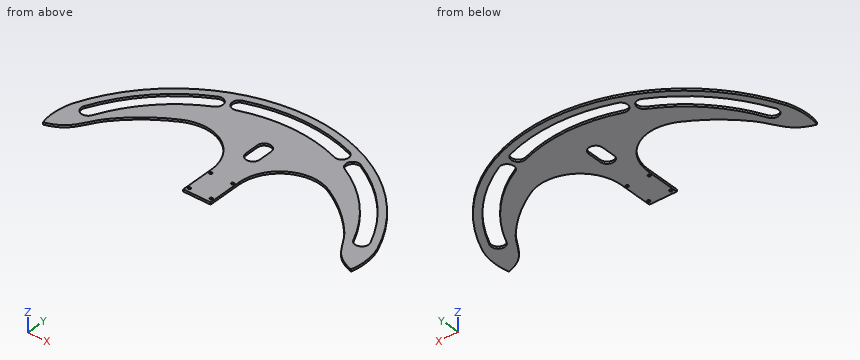
from build123d import *

# Parameters (mm, degrees)
EXTRUDE_2_DEPTH     = 1.6
SKETCH_2_R          = 1
CUT_EXTRUDE_1_DEPTH = 152.556112047


with BuildPart() as part:
    # 草图1 → 凸台-拉伸2 (new body)
    with BuildSketch(Plane.XY):
        with BuildLine():
            Line((-10, 0), (10, 0))
            Line((10, 0), (10, 25))
            ThreePointArc((10, 25), (24.565127337, 50.724787771), (54.117647059, 51.470588235))
            ThreePointArc((54.117647059, 51.470588235), (71.876884233, 39.7703376), (87.177978871, 25))
            add(Edge.make_bspline(
                [(87.177978871, 25), (90.304994573, 21.365241216), (96.247853251, 9.443363931), (103.450341903, 2.775811449), (112.5, 0)],
                knots=[0, 0, 0, 0, 0.44500112, 1, 1, 1, 1], degree=3))
            add(Edge.make_bspline(
                [(111.242977306, 25), (112.528770299, 21.821434652), (115.6681563, 10.742987267), (112.5, 0)],
                knots=[0, 0, 0, 0, 1, 1, 1, 1], degree=3))
            ThreePointArc((111.242977306, 25), (0, 100), (-111.242977306, 25))
            add(Edge.make_bspline(
                [(-111.242977306, 25), (-112.528770299, 21.821434652), (-115.6681563, 10.742987267), (-112.5, 0)],
                knots=[0, 0, 0, 0, 1, 1, 1, 1], degree=3))
            add(Edge.make_bspline(
                [(-87.177978871, 25), (-90.304994573, 21.365241216), (-96.247853251, 9.443363931), (-103.450341903, 2.775811449), (-112.5, 0)],
                knots=[0, 0, 0, 0, 0.44500112, 1, 1, 1, 1], degree=3))
            ThreePointArc((-87.177978871, 25), (-71.876884233, 39.7703376), (-54.117647059, 51.470588235))
            ThreePointArc((-54.117647059, 51.470588235), (-24.565127337, 50.724787771), (-10, 25))
            Line((-10, 25), (-10, 0))
        make_face()
        with BuildLine():
            Line((5, 59.658560997), (5, 49.658560997))
            ThreePointArc((5, 49.658560997), (0, 44.658560997), (-5, 49.658560997))
            Line((-5, 49.658560997), (-5, 59.658560997))
            ThreePointArc((-5, 59.658560997), (0, 64.658560997), (5, 59.658560997))
        make_face(mode=Mode.SUBTRACT)
        with BuildLine():
            ThreePointArc((-52.279803763, 82.046105896), (-83.1008003, 58.999003788), (-104.559607526, 27.051823387))
            ThreePointArc((-104.559607526, 27.051823387), (-102.051823387, 20.440392474), (-95.440392474, 22.948176613))
            ThreePointArc((-95.440392474, 22.948176613), (-75.853125153, 52.10906874), (-47.720196237, 73.146107064))
            ThreePointArc((-47.720196237, 73.146107064), (-45.550000584, 79.875910243), (-52.279803763, 82.046105896))
        make_face(mode=Mode.SUBTRACT)
        with BuildLine():
            ThreePointArc((52.279803763, 82.046105896), (83.1008003, 58.999003788), (104.559607526, 27.051823387))
            ThreePointArc((104.559607526, 27.051823387), (102.051823387, 20.440392474), (95.440392474, 22.948176613))
            ThreePointArc((95.440392474, 22.948176613), (75.853125153, 52.10906874), (47.720196237, 73.146107064))
            ThreePointArc((47.720196237, 73.146107064), (45.550000584, 79.875910243), (52.279803763, 82.046105896))
        make_face(mode=Mode.SUBTRACT)
        with BuildLine():
            ThreePointArc((39.209852822, 87.74587255), (0, 94.658560997), (-39.209852822, 87.74587255))
            ThreePointArc((-39.209852822, 87.74587255), (-42.198553323, 81.337466405), (-35.790147178, 78.348765905))
            ThreePointArc((-35.790147178, 78.348765905), (0, 84.658560997), (35.790147178, 78.348765905))
            ThreePointArc((35.790147178, 78.348765905), (42.198553323, 81.337466405), (39.209852822, 87.74587255))
        make_face(mode=Mode.SUBTRACT)
    extrude(amount=EXTRUDE_2_DEPTH)

    # 草图2 → 切除-拉伸1 (cut, through all)
    with BuildSketch(Plane.XY.offset(1.6)):
        with Locations((-8, 3)):
            Circle(SKETCH_2_R)
        with Locations(Location((8, 3, 0), (0, 0, 180))):
            Circle(SKETCH_2_R)
        with Locations((-8, 22)):
            Circle(SKETCH_2_R)
        with Locations(Location((8, 22, 0), (0, 0, 180))):
            Circle(SKETCH_2_R)
    extrude(amount=-CUT_EXTRUDE_1_DEPTH, mode=Mode.SUBTRACT)


solid = part.part
Could you check a few things on this model? Use its own coordinates, in mm. Give positions to 0.01 mm unless a question says otherwise; leave off trailing zeros. Order: outer loops, then holes, each group sorted by start corner. A loop starts at its lowest first (then second) coordinate and runs counter-clockwise, first axis right, second up. Notation, with made-up numbers: (19.25, -1) -> (47.25, -1) arc R20 cw to (47.25, 29) -> close; hole circle Ø2 at (41, 49.25). An arc over 180 degrees is marked (long way). Answer in a Markdown table with one row per item. Add a question column.
Item 1: Please list where these lines run through material, in increasing order: probe 1 along X at (y, z) = (5, 0.6); probe 2 along Y at (x, z) = (-8, 0.95); probe 3 along X at (y, z) = (50, 0.45).
Item 2: Imagine slicing it at A-A (x = 0). List the corners of the cut face in (y, z) for me.
Item 3: I'm going to push flat-ended pins straight in: P1, Ø12, axis at x = -32, y = 89, coming from the +Z side; P2, Ø0.8, axis at y = 17.5, z = 1, coming from the -X side. Where does each tip first touch, or does it pass through?
Item 4: Imagine slicing it at C-C (y = 34). List the corners of the cut face in (x, z) for me, and give its area (3 significant figures).
Item 5: Imagine slicing it at D-D (z = 1.15). Count the separate pieces of the cut face and the enclosed holes in it, and give its area (3 significant figures).
Item 6: Imagine slicing it at B-B (x = -50). List the corners of the cut face in (y, z) for me.
Result:
| question | item | result |
|---|---|---|
| 1 | probe 1 | -113.55 to -102.06, -10 to 10, 102.06 to 113.55 |
| 1 | probe 2 | 0 to 2, 4 to 21, 23 to 84.35, 94.38 to 99.73 |
| 1 | probe 3 | -97.47 to -90.81, -77.8 to -56.79, -23.42 to -5, 5 to 23.42, 56.79 to 77.8, 90.81 to 97.47 |
| 2 | outline | (0, 0) -> (44.66, 0) -> (44.66, 1.6) -> (0, 1.6) -> close; (64.66, 0) -> (84.66, 0) -> (84.66, 1.6) -> (64.66, 1.6) -> close; (94.66, 0) -> (100, 0) -> (100, 1.6) -> (94.66, 1.6) -> close |
| 3 | P1 | z = 1.6 |
| 3 | P2 | x = -113.29 |
| 4 | outline | (-107.16, 0) -> (-101.15, 0) -> (-101.15, 1.6) -> (-107.16, 1.6) -> close; (-89.65, 0) -> (-78.54, 0) -> (-78.54, 1.6) -> (-89.65, 1.6) -> close; (-11.38, 0) -> (11.38, 0) -> (11.38, 1.6) -> (-11.38, 1.6) -> close; (78.54, 0) -> (89.65, 0) -> (89.65, 1.6) -> (78.54, 1.6) -> close; (101.15, 0) -> (107.16, 0) -> (107.16, 1.6) -> (101.15, 1.6) -> close |
| 4 | area | 91.2 mm2 |
| 5 | separate pieces | 1 |
| 5 | enclosed holes | 8 |
| 5 | area | 7,520 mm2 |
| 6 | outline | (53.28, 0) -> (71.94, 0) -> (71.94, 1.6) -> (53.28, 1.6) -> close; (82.6, 0) -> (89.09, 0) -> (89.09, 1.6) -> (82.6, 1.6) -> close |
